from build123d import *

# Parameters (mm, degrees)
ESBO_O1_R                = 16
RESSALTO_EXTRUS_O1_DEPTH = 4
ESBO_O2_R                = 27
ESBO_O2_R_2              = 24
RESSALTO_EXTRUS_O2_DEPTH = 9
ESBO_O4_R                = 2
CORTE_EXTRUS_O1_DEPTH    = 4
RESSALTO_EXTRUS_O3_START = 9
RESSALTO_EXTRUS_O3_DEPTH = 9
NERVURA4_REACH           = 202.547
ESBO_O8_WALLS_W          = 5
ESBO_O8_WALLS_H          = 505.093505308
ESBO_O9_R                = 1.2
ESBO_O9_W                = 4
ESBO_O9_H                = 10
ESBO_O9_W_2              = 20
ESBO_O9_H_2              = 6
CORTE_EXTRUS_O2_DEPTH    = 4


with BuildPart() as part:
    # Esboço1 → Ressalto-extrusão1 (new body)
    with BuildSketch(Plane.XY):
        with BuildLine():
            Line((45, 0), (45, 150))
            ThreePointArc((45, 150), (0, 195), (-45, 150))
            Line((-45, 150), (-45, 0))
            ThreePointArc((-45, 0), (0, -45), (45, 0))
        make_face()
        Circle(ESBO_O1_R, mode=Mode.SUBTRACT)
        with BuildLine():
            Line((12, 156), (12, 144))
            ThreePointArc((12, 144), (0, 132), (-12, 144))
            Line((-12, 144), (-12, 156))
            ThreePointArc((-12, 156), (0, 168), (12, 156))
        make_face(mode=Mode.SUBTRACT)
        with BuildLine():
            Line((14.49, 159.99), (14.49, 171.99))
            ThreePointArc((14.49, 171.99), (15.99, 173.49), (17.49, 171.99))
            Line((17.49, 171.99), (17.49, 159.99))
            ThreePointArc((17.49, 159.99), (15.99, 158.49), (14.49, 159.99))
        make_face(mode=Mode.SUBTRACT)
        with BuildLine():
            Line((-17.49, 159.99), (-17.49, 171.99))
            ThreePointArc((-17.49, 171.99), (-15.99, 173.49), (-14.49, 171.99))
            Line((-14.49, 171.99), (-14.49, 159.99))
            ThreePointArc((-14.49, 159.99), (-15.99, 158.49), (-17.49, 159.99))
        make_face(mode=Mode.SUBTRACT)
        with BuildLine():
            Line((14.49, 128.01), (14.49, 140.01))
            ThreePointArc((14.49, 140.01), (15.99, 141.51), (17.49, 140.01))
            Line((17.49, 140.01), (17.49, 128.01))
            ThreePointArc((17.49, 128.01), (15.99, 126.51), (14.49, 128.01))
        make_face(mode=Mode.SUBTRACT)
        with BuildLine():
            Line((-17.49, 128.01), (-17.49, 140.01))
            ThreePointArc((-17.49, 140.01), (-15.99, 141.51), (-14.49, 140.01))
            Line((-14.49, 140.01), (-14.49, 128.01))
            ThreePointArc((-14.49, 128.01), (-15.99, 126.51), (-17.49, 128.01))
        make_face(mode=Mode.SUBTRACT)
    extrude(amount=RESSALTO_EXTRUS_O1_DEPTH)

    # Esboço2 → Ressalto-extrusão2 (add)
    with BuildSketch(Plane.XY):
        Circle(ESBO_O2_R)
        Circle(ESBO_O2_R_2, mode=Mode.SUBTRACT)
    extrude(amount=-RESSALTO_EXTRUS_O2_DEPTH)

    # Esboço4 → Corte-extrusão1 (cut)
    with BuildSketch(Plane.XY.offset(4)):
        with Locations((-37, 150)):
            Circle(ESBO_O4_R)
        with Locations((-37, 100)):
            Circle(ESBO_O4_R)
        with Locations((-37, 50)):
            Circle(ESBO_O4_R)
        with Locations((-37, 0)):
            Circle(ESBO_O4_R)
        with Locations((-20.397134603, 180.87)):
            Circle(ESBO_O4_R)
        with Locations((-20.397134603, -30.87)):
            Circle(ESBO_O4_R)
        with Locations((20.397134603, -30.87)):
            Circle(ESBO_O4_R)
        with Locations((20.397134603, 180.87)):
            Circle(ESBO_O4_R)
        with Locations((37, 0)):
            Circle(ESBO_O4_R)
        with Locations((37, 50)):
            Circle(ESBO_O4_R)
        with Locations((37, 100)):
            Circle(ESBO_O4_R)
        with Locations((37, 150)):
            Circle(ESBO_O4_R)
    extrude(amount=-CORTE_EXTRUS_O1_DEPTH, mode=Mode.SUBTRACT)

    # Esboço6 → Ressalto-extrusão3 (add)
    with BuildSketch(Plane(origin=(0, 0, 0), x_dir=(-1, 0, 0), z_dir=(0, 0, -1)).offset(RESSALTO_EXTRUS_O3_START)):
        with BuildLine():
            Line((-14, 143), (-14, 157))
            ThreePointArc((-14, 157), (0, 171), (14, 157))
            Line((14, 157), (14, 143))
            ThreePointArc((14, 143), (0, 129), (-14, 143))
        make_face()
        with BuildLine():
            Line((-12, 144), (-12, 156))
            ThreePointArc((-12, 156), (0, 168), (12, 156))
            Line((12, 156), (12, 144))
            ThreePointArc((12, 144), (0, 132), (-12, 144))
        make_face(mode=Mode.SUBTRACT)
    extrude(amount=-RESSALTO_EXTRUS_O3_DEPTH)

    # Esboço8 walls → Nervura4 (add, up to next)
    with BuildSketch(Plane(origin=(0, 0, -9), x_dir=(-1, 0, 0), z_dir=(0, 0, -1)), mode=Mode.PRIVATE) as nervura4_sk1:
        with Locations((0, 78)):
            Rectangle(ESBO_O8_WALLS_W, ESBO_O8_WALLS_H)
    nervura4_tool1 = extrude(nervura4_sk1.sketch, amount=-NERVURA4_REACH, mode=Mode.PRIVATE) - part.part
    add(nervura4_tool1.solids().sort_by_distance((0, 78, -9))[0])

    # Esboço9 → Corte-extrusão2 (cut)
    with BuildSketch(Plane(origin=(0, 0, 0), x_dir=(-1, 0, 0), z_dir=(0, 0, -1))):
        with Locations((29.032258065, 27.515958854)):
            Circle(ESBO_O9_R)
        with Locations((34.10505047, 35.548192492)):
            Circle(ESBO_O9_R)
        with Locations((32.10505047, 16.515958854)):
            Rectangle(ESBO_O9_W, ESBO_O9_H)
        with Locations((-0.034362558, 175)):
            Rectangle(ESBO_O9_W_2, ESBO_O9_H_2)
        with Locations((-18, 40.548192492)):
            Rectangle(ESBO_O9_W, ESBO_O9_H)
    extrude(amount=-CORTE_EXTRUS_O2_DEPTH, mode=Mode.SUBTRACT)


solid = part.part
Geometry check sheet. Reference: the model listing, model coordinates, mm. A direction names the side the tool comes from. Give positions to 0.01 mm unless a question says otherwise; leave off trailing zeros. Order: outer loops, then holes, each group sorted by start corner. A loop starts at its lowest first (then second) coordinate and runs counter-clockwise, first axis right, second up.
1) Gauge pin test, flat ends, axial feed: pin 1 (1.2 mm diameter, centred on y = 174, z = 1, fed in from -X); pin 2 (5 mm diameter, centred on x = -28.5, y = 26.5, fed in from -Z); pin 3 (5 mm diameter, centred on x = 21.5, z = -1.5, fed in from +Y); pin 4 (4.5 mm diameter, centred on x = -20.4, y = 180.87, fed in from +Z). Record the tip position at first contact, or that the pin passes through.
Results are:
pin 1: stops at x = -38.44
pin 2: stops at z = 0
pin 3: stops at y = 190.56
pin 4: stops at z = 4
2) Cross-section at B-B (y = 117.5). Record the boundary of the cut face in (x, z).
Results are:
outline: (-45, 0) - (-2.5, 0) - (-2.5, -9) - (2.5, -9) - (2.5, 0) - (45, 0) - (45, 4) - (-45, 4) - close
3) Cross-section at A-A (z = -2.5). Record the boundary of the cut face in (x, y).
Results are:
outline: (-14, 143) arc R14 ccw to (-2.5, 129.23) - (-2.5, 26.88) arc R27 ccw (long way) to (2.5, 26.88) - (2.5, 129.23) arc R14 ccw to (14, 143) - (14, 157) arc R14 ccw to (-14, 157) - close; hole circle Ø48 at (0, 0); hole (-12, 144) arc R12 ccw to (12, 144) - (12, 156) arc R12 ccw to (-12, 156) - close
4) Material ranges on probe 1 along Y at (x, z) = (37, 2.5); probe 2 along Y at (x, z) = (-8, -7); probe 3 along X at (y, z) = (47, -2), recorded low to high.
Results are:
probe 1: y = -25.61 to -2, 2 to 48, 52 to 98, 102 to 148, 152 to 175.61
probe 2: y = -25.79 to -22.63, 22.63 to 25.79, 131.51 to 135.06, 164.94 to 168.49
probe 3: x = -2.5 to 2.5
5) Tool access check on faces 1 (the cylindrical face through (10.659, 133.924, -4.563)), 2 (the flat face through (12, 150, -3)), 3 (the cylindrical face through (-23.977, 1.055, -4.437)). Record the directions out of +Z, -Z, +X, -X, +Y, -Y that give a thin tool (end or side, any length) a straight path to the whole face; none if there is none.
Results are:
face 1: -Z, +X
face 2: +Z, -Z
face 3: -Z
6) Draft check along X on faces 4 (the cylindrical face through (0, 171, -5)), 5 (the flat face through (14.49, 134, 2)), 6 (the cylindrical face through (37, 102, 2)), 7 (the flat face through (9, 77, 0)). Enter one of: released by +X, released by -X, zero draft, split by the parting line, or undercut.
Results are:
face 4: split by the parting line
face 5: undercut
face 6: undercut
face 7: zero draft
